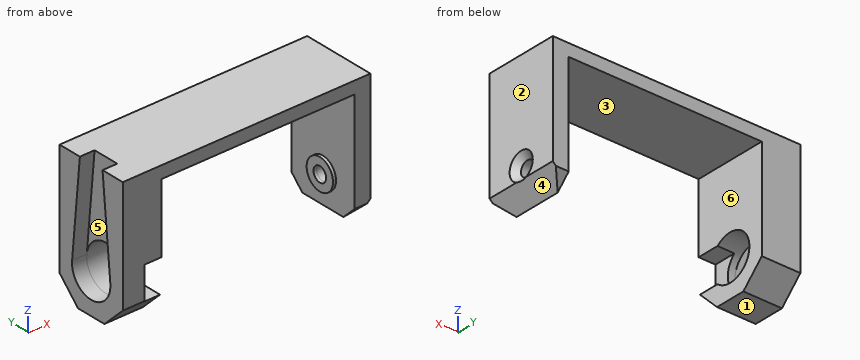
```python
from build123d import *

# Parameters (mm, degrees)
SKETCH1_W                                       = 40.4
SKETCH1_H                                       = 12
BOSS_EXTRUDE1_DEPTH                             = 22
CUT_EXTRUDE1_REACH                              = 34.188
SKETCH2_W                                       = 31.5
SKETCH2_H                                       = 20
CUT_EXTRUDE2_REACH                              = 48.391
SKETCH4_R                                       = 0.9
CHAMFER1_SIZE                                   = 3.5
CSK_FOR_M2_FLAT_HEAD_MACHINE_SCREW1_D           = 2.4
CSK_FOR_M2_FLAT_HEAD_MACHINE_SCREW1_DEPTH       = 12.7
CSK_FOR_M2_FLAT_HEAD_MACHINE_SCREW1_CSINK_D     = 4.4
CSK_FOR_M2_FLAT_HEAD_MACHINE_SCREW1_CSINK_ANGLE = 90
CSK_FOR_M2_FLAT_HEAD_MACHINE_SCREW1_TIP         = 0.721032743
CHAMFER2_SIZE                                   = 4
BOSS_EXTRUDE2_START                             = 0.5
SKETCH20_R                                      = 2.5
SKETCH20_R_2                                    = 1.2
BOSS_EXTRUDE2_DEPTH                             = 0.5
CUT_EXTRUDE3_DEPTH                              = 2.4
SKETCH23_R                                      = 3.65
CUT_EXTRUDE4_DEPTH                              = 22.4
SKETCH24_W                                      = 5.5
SKETCH24_H                                      = 5.5
CUT_EXTRUDE5_DEPTH                              = 22.4


with BuildPart() as part:
    # Sketch1 → Boss-Extrude1 (new body)
    with BuildSketch(Plane.XY):
        Rectangle(SKETCH1_W, SKETCH1_H)
    extrude(amount=BOSS_EXTRUDE1_DEPTH)

    # Sketch2 → Cut-Extrude1 (cut, up to next)
    with BuildSketch(Plane(origin=(0, 6, 0), x_dir=(1, 0, 0), z_dir=(0, 1, 0)), mode=Mode.PRIVATE) as cut_extrude1_sk1:
        with Locations((1.85, -10)):
            Rectangle(SKETCH2_W, SKETCH2_H)
    cut_extrude1_tool1 = extrude(cut_extrude1_sk1.sketch, amount=-CUT_EXTRUDE1_REACH, mode=Mode.PRIVATE) & part.part
    add(cut_extrude1_tool1.solids().sort_by_distance((1.85, 6, 10))[0], mode=Mode.SUBTRACT)

    # Sketch4 → Cut-Extrude2 (cut, up to next)
    with BuildSketch(Plane(origin=(20.2, 0, 0), x_dir=(0, 0, -1), z_dir=(1, 0, 0)), mode=Mode.PRIVATE) as cut_extrude2_sk1:
        with Locations((-6, 0)):
            Circle(SKETCH4_R)
    cut_extrude2_tool1 = extrude(cut_extrude2_sk1.sketch, amount=-CUT_EXTRUDE2_REACH, mode=Mode.PRIVATE) & part.part
    add(cut_extrude2_tool1.solids().sort_by_distance((20.2, 0, 6))[0], mode=Mode.SUBTRACT)

    # Chamfer1
    chamfer1_edges = [part.edges().sort_by_distance(p)[0] for p in [
        (-17.05, -6, 0),
        (-17.05, 6, 0),
        (18.9, -6, 0),
        (18.9, 6, 0),
    ]]
    chamfer(chamfer1_edges, length=CHAMFER1_SIZE)

    # CSK for M2 Flat Head Machine Screw1
    with Locations(Plane(origin=(20.2, 0, 0), x_dir=(0, 0, -1), z_dir=(1, 0, 0))):
        with Locations((-6, 0)):
            CounterSinkHole(CSK_FOR_M2_FLAT_HEAD_MACHINE_SCREW1_D / 2, CSK_FOR_M2_FLAT_HEAD_MACHINE_SCREW1_CSINK_D / 2, depth=CSK_FOR_M2_FLAT_HEAD_MACHINE_SCREW1_DEPTH, counter_sink_angle=CSK_FOR_M2_FLAT_HEAD_MACHINE_SCREW1_CSINK_ANGLE)
            with Locations((0, 0, -(CSK_FOR_M2_FLAT_HEAD_MACHINE_SCREW1_DEPTH + CSK_FOR_M2_FLAT_HEAD_MACHINE_SCREW1_TIP / 2))):  # 118° drill point
                Cone(0, CSK_FOR_M2_FLAT_HEAD_MACHINE_SCREW1_D / 2, CSK_FOR_M2_FLAT_HEAD_MACHINE_SCREW1_TIP, mode=Mode.SUBTRACT)

    # Chamfer2
    # the kernel refuses this chamfer: 4 mm, written as the material it takes off along each edge
    with BuildSketch(Plane(origin=(20.2, 12.786731952, 0), x_dir=(-0.9996219169112968, 0, -0.027495876610586365), z_dir=(0, -1, 0))) as chamfer2_piece_1:
        Polygon((CHAMFER2_SIZE * 0.999621916911, -CHAMFER2_SIZE * 0.0274958766106), (-CHAMFER2_SIZE * 0.0274958766106, -CHAMFER2_SIZE * 0.999621916911), (0, 0), align=None)
    extrude(amount=25.573463904, mode=Mode.SUBTRACT)

    # Sketch20 → Boss-Extrude2 (add)
    with BuildSketch(Plane.ZY.offset(-17.6).offset(BOSS_EXTRUDE2_START)):
        with Locations(Location((6, 0, 0), (0, 0, 180))):
            Circle(SKETCH20_R)
        with Locations(Location((6, 0, 0), (0, 0, 180))):
            Circle(SKETCH20_R_2, mode=Mode.SUBTRACT)
    extrude(amount=-BOSS_EXTRUDE2_DEPTH)

    # Sketch5 → Cut-Extrude3 (cut)
    with BuildSketch(Plane.ZY.offset(20.2)):
        with BuildLine():
            Line((6.343920973, 3.633760912), (22.64787234, 2.090656963))
            ThreePointArc((22.64787234, 2.090656963), (24.55, 0), (22.64787234, -2.090656963))
            Line((22.64787234, -2.090656963), (6.343920973, -3.633760912))
            ThreePointArc((6.343920973, -3.633760912), (2.35, 0), (6.343920973, 3.633760912))
        make_face()
    extrude(amount=-CUT_EXTRUDE3_DEPTH, mode=Mode.SUBTRACT)

    # Sketch23 → Cut-Extrude4 (cut)
    with BuildSketch(Plane.ZY.offset(17.8)):
        with Locations((6, 0)):
            Circle(SKETCH23_R)
    extrude(amount=-CUT_EXTRUDE4_DEPTH, mode=Mode.SUBTRACT)

    # Sketch24 → Cut-Extrude5 (cut)
    with BuildSketch(Plane(origin=(0, 0, 0), x_dir=(-1, 0, 0), z_dir=(0, -1, 0))):
        with Locations((13.9, -6)):
            Rectangle(SKETCH24_W, SKETCH24_H)
    extrude(amount=CUT_EXTRUDE5_DEPTH, mode=Mode.SUBTRACT)


solid = part.part
```
For this review, take the finished solid that the model builds, in its own axes (mm). Face numbers are marked on the shaded views. A direction names the side the tool comes from. Give positions to 0.01 mm unless a question says otherwise; leave off trailing zeros. Order: outer loops, then holes, each group sorted by start corner. A loop starts at its lowest first (then second) coordinate and runs counter-clockwise, first axis right, second up.
1) Wall thickness on line 1 (X direction, y = 3.5, z = 13); line 2 (Y direction, x = -19, z = 6); line 3 (Z direction, x = -15.9, y = 0): over which ranges is each line inside the solid? List them lowest first.
2) For the marked faces 4, 5 and 6, list the 3-axis set-ups (+Z, -Z, +X, -X, +Y, -Y) from which the entire face can be reached by the end or side of a thin tool; tool diameter is ignored.
3) Take a section at C-C (y = 5). Give the boundary of the cut face in (x, z).
4) Take a section at B-B (z = 11.5). Give the boundary of the cut face in (x, y), then the cut area to 3 significant figures.
5) Take a section at A-A (y = 0). Give the boundary of the cut face in (x, z).
6) Take a section at D-D (x = 12). Give the boundary of the cut face in (y, z), then the cut area to 3 significant figures.
7) The part is to be moulded in two halves that separate along X. For the marked faces 1, 2 and 3, say which applies: released by +X, released by -X, zero draft, split by the parting line, or undercut.
8) Insertion check: pin 1 (6.5 mm diameter, centred on y = 0, z = 6, fed in from +X); pin 2 (3 mm diameter, centred on y = 0, z = 6, fed in from -X); pin 3 (3 mm diameter, centred on y = 0, z = 6, fed in from +X); pin 4 (2 mm diameter, centred on y = -1, z = 13, fed in from -X). Each pin has a flat end and moves straight along its axis. Give the tip position at first contact, or say it passes through.
Derived:
1. line 1: x = -20.2 to -13.9, 17.6 to 20.2
1. line 2: y = -6 to -3.65, 3.65 to 6
1. line 3: z = 0 to 2.35, 9.65 to 22
2. face 4: -Z, +X, +Y, -Y
2. face 5: -X
2. face 6: -Z, +Y, -Y
3. outline: (-20.2, 2.5) - (-13.9, 2.5) - (-13.9, 20) - (17.6, 20) - (17.6, 2.5) - (18.7, 2.5) - (20.2, 4) - (20.2, 22) - (-20.2, 22) - close
4. outline: (-20.2, -6) - (-13.9, -6) - (-13.9, 6) - (-20.2, 6) - (-20.2, 3.15) - (-17.8, 3.15) - (-17.8, -3.15) - (-20.2, -3.15) - close; (17.6, -6) - (20.2, -6) - (20.2, 6) - (17.6, 6) - close
4. area: 91.7 mm2
5. outline: (-20.2, 0) - (-13.9, 0) - (-13.9, 2.35) - (-20.2, 2.35) - close; (-17.8, 9.65) - (-13.9, 9.65) - (-13.9, 20) - (17.6, 20) - (17.6, 8.5) - (17.1, 8.5) - (17.1, 7.2) - (19.2, 7.2) - (20.2, 8.2) - (20.2, 22) - (-17.8, 22) - close; (17.1, 3.5) - (17.6, 3.5) - (17.6, 1.4) - (20.1, 3.9) - (19.2, 4.8) - (17.1, 4.8) - close
6. outline: (-6, 20) - (6, 20) - (6, 22) - (-6, 22) - close
6. area: 24.0 mm2
7. face 1: zero draft
7. face 2: released by +X
7. face 3: undercut
8. pin 1: stops at x = 20.2
8. pin 2: stops at x = 17.1
8. pin 3: stops at x = 19.5
8. pin 4: stops at x = -17.8
